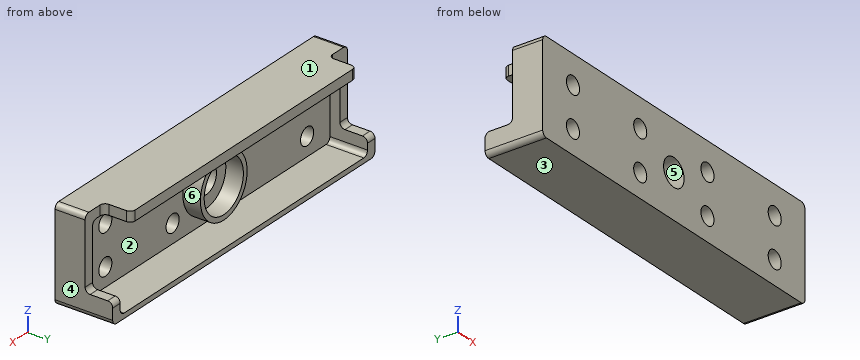
from build123d import *

# Parameters (mm, degrees)
SKETCH1_W           = 35.1
SKETCH1_H           = 18.5
BOSS_EXTRUDE1_DEPTH = 11.5
SKETCH7_W           = 33.1
SKETCH7_H           = 15.5
CUT_EXTRUDE5_DEPTH  = 7.5
SKETCH2_R           = 1.75
CUT_EXTRUDE1_DEPTH  = 39.076534769
SKETCH4_W           = 14.25
SKETCH4_H           = 5.5
CUT_EXTRUDE3_DEPTH  = 5
SKETCH5_R           = 2.75
CUT_EXTRUDE4_DEPTH  = 39.076534769
SKETCH6_R           = 6.25
SKETCH6_R_2         = 5.25
BOSS_EXTRUDE2_DEPTH = 3.5
FILLET3_R           = 1
FILLET6_R           = 1


with BuildPart() as part:
    # Sketch1 → Boss-Extrude1 (new body)
    with BuildSketch(Plane(origin=(0, 0, 0), x_dir=(1, 0, 0), z_dir=(0, 1, 0))):
        with Locations((-17.55, 0)):
            Rectangle(SKETCH1_W, SKETCH1_H)
    extrude(amount=BOSS_EXTRUDE1_DEPTH)

    # Sketch7 → Cut-Extrude5 (cut)
    with BuildSketch(Plane(origin=(0, 11.5, 0), x_dir=(1, 0, 0), z_dir=(0, 1, 0))):
        with Locations((-16.55, 0.5)):
            Rectangle(SKETCH7_W, SKETCH7_H)
    extrude(amount=-CUT_EXTRUDE5_DEPTH, mode=Mode.SUBTRACT)

    # Sketch2 → Cut-Extrude1 (cut, through all)
    with BuildSketch(Plane(origin=(0, 0, 0), x_dir=(-1, 0, 0), z_dir=(0, 1, 0))):
        with Locations(Location((27, 3.5, 0), (0, 0, 270))):
            Circle(SKETCH2_R)
        with Locations(Location((9, 3.5, 0), (0, 0, 270))):
            Circle(SKETCH2_R)
        with Locations(Location((27, -4.5, 0), (0, 0, 270))):
            Circle(SKETCH2_R)
        with Locations(Location((9, -4.5, 0), (0, 0, 270))):
            Circle(SKETCH2_R)
    extrude(amount=CUT_EXTRUDE1_DEPTH, mode=Mode.SUBTRACT)

    # Sketch4 → Cut-Extrude3 (cut)
    with BuildSketch(Plane.ZY.offset(35.1)):
        with Locations((2.125, 8.75)):
            Rectangle(SKETCH4_W, SKETCH4_H)
    extrude(amount=-CUT_EXTRUDE3_DEPTH, mode=Mode.SUBTRACT)

    # Mirror1: part across plane


with BuildPart() as part_1:
    add(part.part)
    add(part.part.mirror(Plane(origin=(0, 0, 0), x_dir=(0, 0, 1), z_dir=(1, 0, 0))))

    # Sketch5 → Cut-Extrude4 (cut, through all)
    with BuildSketch(Plane(origin=(0, 0, 0), x_dir=(1, 0, 0), z_dir=(0, 1, 0))):
        with Locations(Location((0, 0.5, 0), (0, 0, 90))):
            Circle(SKETCH5_R)
    extrude(amount=CUT_EXTRUDE4_DEPTH, mode=Mode.SUBTRACT)

    # Sketch6 → Boss-Extrude2 (add)
    with BuildSketch(Plane(origin=(0, 4, 0), x_dir=(1, 0, 0), z_dir=(0, 1, 0))):
        with Locations(Location((0, 0.5, 0), (0, 0, 90))):
            Circle(SKETCH6_R)
        with Locations(Location((0, 0.5, 0), (0, 0, 270))):
            Circle(SKETCH6_R_2, mode=Mode.SUBTRACT)
    extrude(amount=BOSS_EXTRUDE2_DEPTH)

    # Fillet3
    fillet3_edges = [part_1.edges().sort_by_distance(p)[0] for p in [
        (-34.1, 6, -5),
        (-34.1, 11.5, -5),
        (-30.1, 11.5, 8.25),
        (-30.1, 6, 8.25),
        (34.1, 11.5, -5),
        (34.1, 6, -5),
        (30.1, 11.5, 8.25),
        (30.1, 6, 8.25),
    ]]
    fillet(fillet3_edges, radius=FILLET3_R)

    # Fillet6
    fillet6_edges = [part_1.edges().sort_by_distance(p)[0] for p in [
        (-33.1, 7.75, -8.25),
        (-33.1, 5, 7.25),
        (-35.1, 3, 9.25),
        (35.1, 5.75, -9.25),
        (35.1, 3, 9.25),
        (33.1, 7.75, -8.25),
        (33.1, 5, 7.25),
        (-35.1, 5.75, -9.25),
    ]]
    fillet(fillet6_edges, radius=FILLET6_R)


solid = part_1.part
Part model, mm, in its own coordinate system. Face numbers are marked on the shaded views. A direction names the side the tool comes from. Round coordinates to 2 decimals unless told otherwise and drop trailing zeros. Write each loop counter-clockwise with the first axis right and the second up, starting at its lowest first coordinate (ties: lowest second). Pieces come first, ordered by that corner, then holes. Notation, with made-up numbers: M 43.5,30.25 L 94.5,30.25 A25 ccw 94.5,42.25 Z; hole C 26.25,86 d9. An arc over 180 degrees is marked long. Return JSON: item names as keys, results as strings. Group by question number.
(1) Which spindle directions (+Z, -Z, +X, -X, +Y, -Y) get a long thin tool onto all of the face, cutting with end or side? Do the marked faces 5 and 6. Say none if no direction does.
(2) Saw through at B-B on x = -27. Write the cut outline in (y, z), then the cut area to 3 significant figures.
(3) Saw through at A-A on y = 5. Write the cut outline in (x, z).
(4) Drill centre lines: probe 1 along X at (y, z) = (3.75, -4.5); probe 2 along Z at (x, y) = (-9, 2.1); probe 3 along X at (y, z) = (4.5, -0.5). Where is each one in solid material? Low to high.
(5) Two-plate mould, pull along Z, no slides. Class the marked faces 1, 2, 3 and 4: +Z half, -Z half, draft (parallel to the pull), parting line (faces both ways), or undercut.
(6) Pin check, flat tips, straight feed: pin 1 Ø0.6 at (y, z) = (8.5, 8) entering from -X; pin 2 Ø4.5 at (x, z) = (-9, -4.5) entering from +Y; pin 3 Ø1.2 at (x, z) = (-33, 5.5) entering from +Y. Stop position of each tip, or through.
(7) Saw through at D-D on x = 0. Write the cut outline in (y, z), then the cut area to 3 significant figures.
(8) Saw through at C-C on y = 8.5. Write the cut outline in (x, z), then the cut area to 3 significant figures.
Returned:
{
 "1": {"face 5": "+Y, -Y", "face 6": "+Y"},
 "2": {"outline": "M 0,-9.25 L 11.5,-9.25 L 11.5,-8.25 L 4,-8.25 L 4,-6.25 L 0,-6.25 Z; M 0,-2.75 L 4,-2.75 L 4,1.75 L 0,1.75 Z; M 0,5.25 L 4,5.25 L 4,7.25 L 11.5,7.25 L 11.5,9.25 L 0,9.25 Z", "area": "68.5 mm²"},
 "3": {"outline": "M -35.1,-8.25 A1 ccw -34.1,-9.25 L 34.1,-9.25 A1 ccw 35.1,-8.25 L 35.1,8.25 A1 ccw 34.1,9.25 L -34.1,9.25 A1 ccw -35.1,8.25 Z; C 0,-0.5 d12.5; hole M -33.1,-7.25 A1 ccw -32.1,-8.25 L 32.1,-8.25 A1 ccw 33.1,-7.25 L 33.1,6.25 A1 ccw 32.1,7.25 L -32.1,7.25 A1 ccw -33.1,6.25 Z; hole C 0,-0.5 d10.5"},
 "4": {"probe 1": "-35.1 to -28.75, -25.25 to -10.75, -7.25 to 7.25, 10.75 to 25.25, 28.75 to 35.1", "probe 2": "-9.25 to -6.25, -2.75 to 1.75, 5.25 to 9.25", "probe 3": "-35.1 to -33.1, -6.25 to -5.25, 5.25 to 6.25, 33.1 to 35.1"},
 "5": {"face 1": "+Z half", "face 2": "undercut", "face 3": "-Z half", "face 4": "draft"},
 "6": {"pin 1": "x = -30.1", "pin 2": "y = 4", "pin 3": "y = 6"},
 "7": {"outline": "M 0,-9.25 L 11.5,-9.25 L 11.5,-8.25 L 4,-8.25 L 4,-6.75 L 7.5,-6.75 L 7.5,-5.75 L 4,-5.75 L 4,-3.25 L 0,-3.25 Z; M 0,2.25 L 4,2.25 L 4,4.75 L 7.5,4.75 L 7.5,5.75 L 4,5.75 L 4,7.25 L 11.5,7.25 L 11.5,9.25 L 0,9.25 Z", "area": "81.5 mm²"},
 "8": {"outline": "M -35.1,-8.25 A1 ccw -34.1,-9.25 L 34.1,-9.25 A1 ccw 35.1,-8.25 L 35.1,-5 L 33.1,-5 L 33.1,-7.25 A1 cw 32.1,-8.25 L -32.1,-8.25 A1 cw -33.1,-7.25 L -33.1,-5 L -35.1,-5 Z; M -30.1,7.25 L 30.1,7.25 L 30.1,9.25 L -30.1,9.25 Z", "area": "204 mm²"}
}
